Geometry: see drawing. Coordinates: mm, zero at the bounding-box minimum. A direction names the side the tool comes from. Coordinates: 2 decimals unless noted, no trailing zeros. Order: outer loops, then holes, each group sorted by start corner. A loop starts at its lowest first (then second) coordinate and runs counter-clockwise, first axis right, second up.
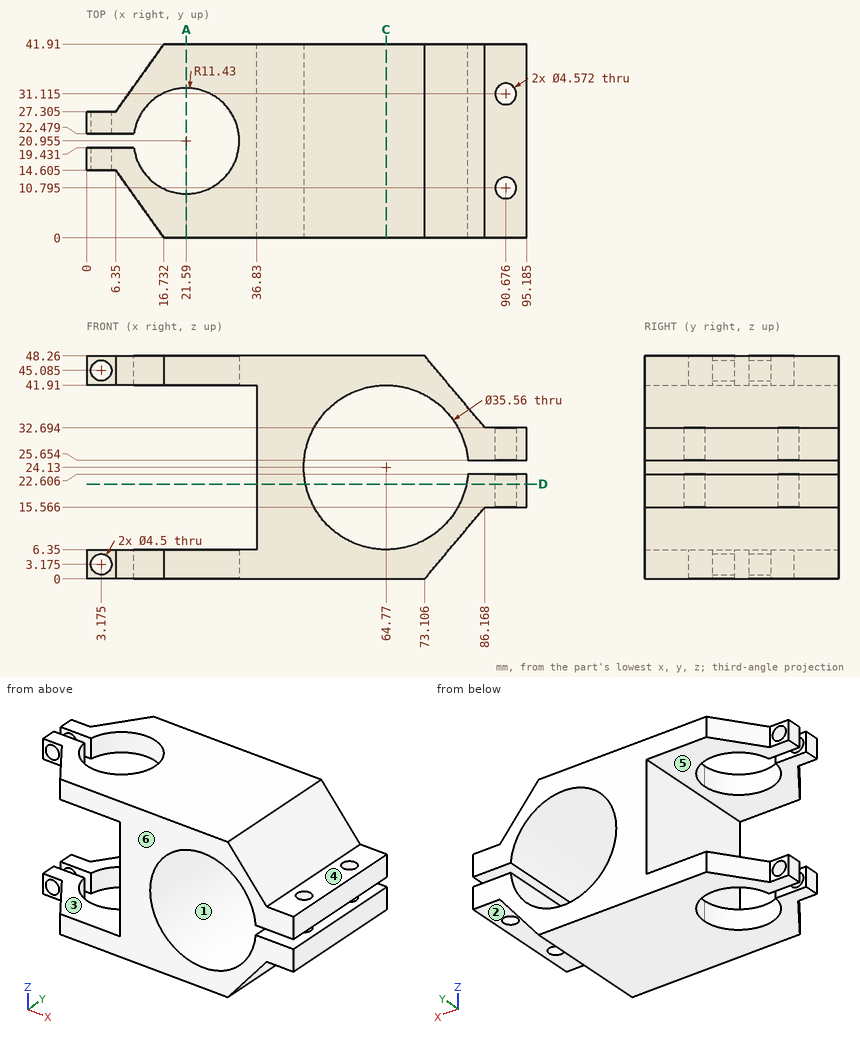
Q1. Material intervals for line 1 along Z through (x, y) = (21.5, 7); line 2 along Z through (x, y) = (49.5, 28.5) (1 decimal); line 3 along X through (y, z) = (31, 46.5) (1 decimal), sorted ascending.
Solutions:
line 1: z = 0 to 6.35, 41.91 to 48.26
line 2: z = 0 to 15, 33.2 to 48.3
line 3: x = 9 to 16.1, 27 to 74.6
Q2. Pull-direction query (Z, two-part tool) for the marked faces 4, 5 and 6; classes: pulls with the +Z half, pulls with the -Z half, needs draft (parallel to the pull), parting line crosses it, or undercut.
Solutions:
face 4: pulls with the +Z half
face 5: undercut
face 6: needs draft
Q3. Section query C-C on x = 64.77. Output: boundary loops of the cut face in (y, z).
Solutions:
outline: (0, 0) - (41.91, 0) - (41.91, 6.35) - (0, 6.35) - close; (0, 41.91) - (41.91, 41.91) - (41.91, 48.26) - (0, 48.26) - close
Q4. Section query D-D on z = 20.5. Output: boundary loops of the cut face in (x, y) (1 decimal).
Solutions:
outline: (36.8, 0) - (47.4, 0) - (47.4, 41.9) - (36.8, 41.9) - close; (82.2, 0) - (95.2, 0) - (95.2, 41.9) - (82.2, 41.9) - close; hole circle Ø4.6 at (90.7, 10.8); hole circle Ø4.6 at (90.7, 31.1)
Q5. Section query A-A on x = 21.59. Give the number of separate pieces and of enclosed holes in the cut face, plus the area to 3 significant figures.
Solutions:
separate pieces: 4
enclosed holes: 0
area: 242 mm2
Q6. Set-up query: the marked faces 1, 2 and 3. Return all of +Z, -Z, +X, -X, +Y, -Y with unobstructed straight access to the full face (end or side cutting, diameter ignored); none if empty.
Solutions:
face 1: +Y, -Y
face 2: -Z, +X, +Y, -Y
face 3: -X, +Y, -Y
Q7. Pin query (flat end, axial travel): P1, Ø5, axis at x = 4, z = 44.5, coming from the -Y side (1 decimal); P2, Ø1.9, axis at x = 7, z = 44.5, coming from the +Y side (1 decimal); P3, Ø7, axis at x = 7.5, z = 3, coming from the +Y side (1 decimal); P4, Ø11, axis at x = 11, y = 18.5, coming from the +Z side. Return the tip coordinate at first contact, or that it passes through.
Solutions:
P1: stops at y = 14.4
P2: stops at y = 29.6
P3: stops at y = 33.8
P4: stops at z = 48.26
